The model under review builds one solid part; all positions refer to its coordinate system, in mm. Face numbers are marked on the shaded views. A direction names the side the tool comes from. Give positions to 0.01 mm unless a question says otherwise; leave off trailing zeros. Loops run counter-clockwise (first coordinate to the right, second up) from the corner with the lowest first, then second, coordinate; pieces in that order, holes last. Notation, with made-up numbers: M 29.25,-8 L 62.25,-8 A15 cw 62.25,10 Z; hole C 38,73 d5. An arc over 180 degrees is marked long. Put each result on its own line as item: value. Start each with the question number.
```python
from build123d import *

# Parameters (mm, degrees)
BOSS_EXTRUDE1_DEPTH = 3.175
FILLET1_R           = 3.175


with BuildPart() as part:
    # Sketch1 → Boss-Extrude1 (new body)
    with BuildSketch(Plane.XY):
        Polygon((9.525, 0), (15.875, 0), (15.875, -3.175), (22.225, -3.175), (22.225, 0), (28.575, 0), (28.575, -3.175), (34.925, -3.175), (34.925, 0), (38.1, 0), (38.1, 28.575), (0, 28.575), (0, 0), (3.175, 0), (3.175, -3.175), (9.525, -3.175), align=None)
    extrude(amount=BOSS_EXTRUDE1_DEPTH)

    # Fillet1
    fillet1_edges = [part.edges().sort_by_distance(p)[0] for p in [
        (0, 28.575, 1.5875),
        (38.1, 28.575, 1.5875),
    ]]
    fillet(fillet1_edges, radius=FILLET1_R)


solid = part.part
```
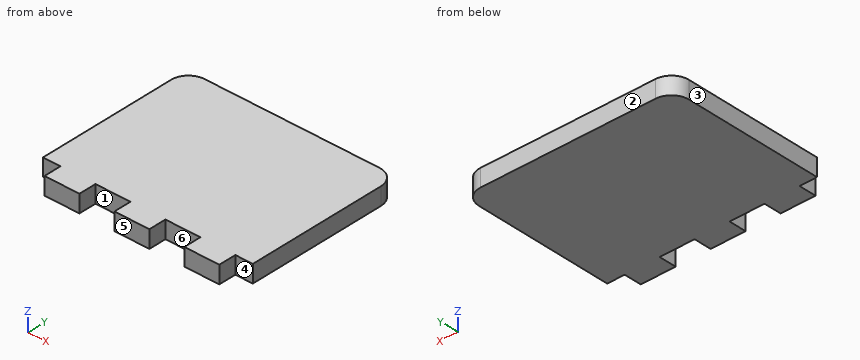
Item 1: Consider section B-B, the plane z = 1.2. Write out the cut boundary in (x, y) (3 decimals), plus the area to 3 significant figures.
Item 2: Consider section D-D, the plane x = 36. Write out the cut boundary in (y, z) (3 decimals), plus the area to 3 significant figures.
Item 3: Draft analysis for pull direction X (two halves, no side actions). For the marked faces 1, 2 and 3, state which applies: +X half, -X half, draft (parallel to the pull), parting line (faces both ways), or undercut.
Item 4: Clearance check with flat-ended pins moving along their axes: pin 1 Ø1 at (x, z) = (14, 2) entering from -Y; pin 2 Ø1 at (y, z) = (-2, 1.5) entering from +X (3 decimals). State where each tip first meets the part, or that it passes through.
Item 5: Tool access review of the marked faces 4, 5 and 6: name each direction out of +Z, -Z, +X, -X, +Y, -Y from which nothing blocks a thin tool from reaching the whole face with its end or side.
Item 6: Consider section A-A, the plane y = -1. Write out the cut boundary in (x, z) (3 decimals), plus the area to 3 significant figures.
Item 7: Consider section C-C, the plane x = 10. Write out the cut boundary in (y, z) (3 decimals), plus the area to 3 significant figures.
Item 8: To check wall thickness, follow L1, parallel to X at y = -2, z = 2.7 (3 decimals); L2, parallel to Y at x = 27.5, z = 2.75 (3 decimals); L3, parallel to X at y = 27.5, z = 1.65. State the ranges of each line that lie inside material, in increasing order. Write a range as [from, to].
Report:
1. outline: M 0,0 L 3.175,0 L 3.175,-3.175 L 9.525,-3.175 L 9.525,0 L 15.875,0 L 15.875,-3.175 L 22.225,-3.175 L 22.225,0 L 28.575,0 L 28.575,-3.175 L 34.925,-3.175 L 34.925,0 L 38.1,0 L 38.1,25.4 A3.175 ccw 34.925,28.575 L 3.175,28.575 A3.175 ccw 0,25.4 Z
1. area: 1,140 mm²
2. outline: M 0,0 L 28.387,0 L 28.387,3.175 L 0,3.175 Z
2. area: 90.1 mm²
3. face 1: undercut
3. face 2: draft
3. face 3: -X half
4. pin 1: y = 0
4. pin 2: x = 34.925
5. face 4: +Z, -Z, +X, -Y
5. face 5: +Z, -Z, +X, -X, -Y
5. face 6: +Z, -Z, -Y
6. outline: M 3.175,0 L 9.525,0 L 9.525,3.175 L 3.175,3.175 Z; M 15.875,0 L 22.225,0 L 22.225,3.175 L 15.875,3.175 Z; M 28.575,0 L 34.925,0 L 34.925,3.175 L 28.575,3.175 Z
6. area: 60.5 mm²
7. outline: M 0,0 L 28.575,0 L 28.575,3.175 L 0,3.175 Z
7. area: 90.7 mm²
8. L1: [3.175, 9.525], [15.875, 22.225], [28.575, 34.925]
8. L2: [0, 28.575]
8. L3: [0.79, 37.31]
